```python
from build123d import *

# Parameters (mm, degrees)
SKETCH1_W                  = 25.4
SKETCH1_H                  = 44.45
BOSS_EXTRUDE1_DEPTH        = 12.7
SKETCH2_W                  = 25.4
SKETCH2_H                  = 19.05
CUT_EXTRUDE1_DEPTH         = 12.7
SKETCH3_R                  = 3.175
CUT_EXTRUDE2_DEPTH         = 37.061067996
F_1_4_CLEARANCE_HOLE1_D    = 6.7564
F_6_32_TAPPED_HOLE1_REACH  = 49.941
F_6_32_TAPPED_HOLE1_BORE_R = 1.35255


with BuildPart() as part:
    # Sketch1 → Boss-Extrude1 (new, symmetric)
    with BuildSketch(Plane.XY):
        Rectangle(SKETCH1_W, SKETCH1_H)
    extrude(amount=BOSS_EXTRUDE1_DEPTH, both=True)

    # Sketch2 → Cut-Extrude1 (cut)
    with BuildSketch(Plane(origin=(0, 0, -12.7), x_dir=(-1, 0, 0), z_dir=(0, 0, -1))):
        with Locations((0, 6.35)):
            Rectangle(SKETCH2_W, SKETCH2_H)
    extrude(amount=-CUT_EXTRUDE1_DEPTH, mode=Mode.SUBTRACT)

    # Sketch3 → Cut-Extrude2 (cut, through all)
    with BuildSketch(Plane.XY.offset(12.7)):
        with Locations((0, -12.7)):
            Circle(SKETCH3_R)
    extrude(amount=-CUT_EXTRUDE2_DEPTH, mode=Mode.SUBTRACT)

    # 1/4 Clearance Hole1 (through all)
    with Locations(Plane(origin=(0, 0, 0), x_dir=(-1, 0, 0), z_dir=(0, 0, -1))):
        with Locations((0, 6.35)):
            Hole(F_1_4_CLEARANCE_HOLE1_D / 2)

    # #6-32 Tapped Hole1 bore → #6-32 Tapped Hole1 (cut, up to next)
    with BuildSketch(Plane(origin=(0, -22.225, 0), x_dir=(-1, 0, 0), z_dir=(0, -1, 0)), mode=Mode.PRIVATE) as f_6_32_tapped_hole1_sk1:
        Circle(F_6_32_TAPPED_HOLE1_BORE_R)
    f_6_32_tapped_hole1_tool1 = extrude(f_6_32_tapped_hole1_sk1.sketch, amount=-F_6_32_TAPPED_HOLE1_REACH, mode=Mode.PRIVATE) & part.part
    add(f_6_32_tapped_hole1_tool1.solids().sort_by_distance((0, -22.225, 0))[0], mode=Mode.SUBTRACT)


solid = part.part
```
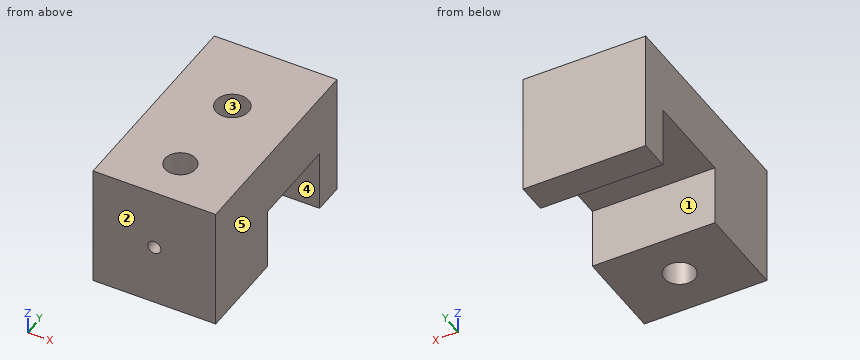
Geometry: final body of the model. Coordinates: model frame, mm. Face numbers are marked on the shaded views. A direction names the side the tool comes from. Coordinates: 2 decimals unless noted, no trailing zeros. Write each loop counter-clockwise with the first axis right and the second up, starting at its lowest first coordinate (ties: lowest second). Pieces come first, ordered by that corner, then holes. Notation, with made-up numbers: M 46.5,-26.75 L 64.5,-26.75 A16 cw 64.5,-3.75 Z; hole C 1.5,37.5 d6. An arc over 180 degrees is marked long. Use CSV: the item, a comma, the result in double quotes. Start each with the question number.
1. Ray query, probe 1 along Y at (x, z) = (0, -5.5) (3 decimals); probe 2 along Y at (x, z) = (0, 4) (3 decimals); probe 3 along Y at (x, z) = (-8.5, -2.25) (3 decimals). Return the intervals inside material, ascending.
2. Mould query, pull axis X, two halves, no side actions, for the marked faces 3, 4 and 5. Classes: pulls with the +X half, pulls with the -X half, needs draft (parallel to the pull), parting line crosses it, or undercut.
3. Reachability of the marked faces 1 and 2 from +Z, -Z, +X, -X, +Y, -Y: full face, straight path, thin tool, end or side. Return the list, or none.
4. Cut plane D-D on x = -9.5. Return the cut outline in (y, z) (3 decimals), plus the area to 3 significant figures.
5. Cut plane A-A on z = -6.25. Return the cut outline in (x, y) (3 decimals).
6. Cut plane B-B on y = -12.7. Return the cut outline in (x, z) (3 decimals), plus the area to 3 significant figures.
7. First-contact query: P1, Ø8, axis at x = 0, y = 6.35, coming from the -Z side. Flat tip, straight axial feed; report the tip coordinate or a pass-through.
8. Cut plane C-C on x = 0. Return the cut outline in (y, z) (3 decimals).
Entries:
1,probe 1,"-22.225 to -15.875, -9.525 to -3.175, 15.875 to 22.225"
1,probe 2,"-22.225 to -15.875, -9.525 to 2.972, 9.728 to 22.225"
1,probe 3,"-22.225 to -3.175, 15.875 to 22.225"
2,face 3,"undercut"
2,face 4,"needs draft"
2,face 5,"pulls with the +X half"
3,face 1,"-Z, +X, -X"
3,face 2,"+Z, -Z, +X, -X, -Y"
4,outline,"M -22.225,-12.7 L -3.175,-12.7 L -3.175,0 L 15.875,0 L 15.875,-12.7 L 22.225,-12.7 L 22.225,12.7 L -22.225,12.7 Z"
4,area,"887 mm²"
5,outline,"M -12.7,-22.225 L 12.7,-22.225 L 12.7,-3.175 L -12.7,-3.175 Z; M -12.7,15.875 L 12.7,15.875 L 12.7,22.225 L -12.7,22.225 Z; hole C 0,-12.7 d6.35"
6,outline,"M -12.7,-12.7 L -3.175,-12.7 L -3.175,12.7 L -12.7,12.7 Z; M 3.175,-12.7 L 12.7,-12.7 L 12.7,12.7 L 3.175,12.7 Z"
6,area,"484 mm²"
7,P1,"z = 0"
8,outline,"M -22.225,-12.7 L -15.875,-12.7 L -15.875,-1.353 L -22.225,-1.353 Z; M -22.225,1.353 L -15.875,1.353 L -15.875,12.7 L -22.225,12.7 Z; M -9.525,-12.7 L -3.175,-12.7 L -3.175,0 L 2.972,0 L 2.972,12.7 L -9.525,12.7 Z; M 9.728,0 L 15.875,0 L 15.875,-12.7 L 22.225,-12.7 L 22.225,12.7 L 9.728,12.7 Z"
